Autodesk Inventor part; units mm, degrees
ref_plane "YZ Plane" through (0, 0, 0) normal (1, 0, 0) x (0, 1, 0)
ref_plane "XZ Plane" through (0, 0, 0) normal (0, 1, 0) x (-1, 0, 0)
ref_plane "XY Plane" through (0, 0, 0) normal (0, 0, 1) x (1, 0, 0)
sketch "Boceto1" plane through (0, 0, 0) normal (1, 0, 0) x (0, 1, 0)
  line L0 (-16, 16) -> (16, 16)
  line L1 (16, 16) -> (16, -16)
  line L2 (16, -16) -> (-16, -16)
  line L3 (-16, -16) -> (-16, 16)
  line L4 (-16, 16) -> (16, -16) construction
  line L5 (16, 16) -> (-16, -16) construction
  line L6 (17, 17) -> (-17, 17)
  line L7 (-17, 17) -> (-17, -17)
  line L8 (-17, -17) -> (17, -17)
  line L9 (17, -17) -> (17, 17)
  line L10 (17, 17) -> (-17, -17) construction
  line L11 (-17, 17) -> (17, -17) construction
  point P0 (0, 0)
  dimension "d0" = 32
  dimension "d1" = 32
  dimension "d2" = 34
  dimension "d3" = 34
extrude "Extrusión1" add sketch "Boceto1" along normal blind 100
sketch "Boceto5" plane through (0, 17, 17) normal (0, 1, 0) x (1, 0, 0)
  line L0 (100, 1) -> (100, 33)
  line L1 (100, 17) -> (88.5, 17) construction
  line L2 (88.5, 17) -> (82, 17) construction
  line L3 (82, 17) -> (82, 30.5) construction
  circle A0 centre (82, 30.5) radius 1.25
  circle A1 centre (74, 30.5) radius 1.25
  line L4 (80.5, 17) -> (74, 17) construction
  circle A2 centre (66, 30.5) radius 1.25
  line L5 (72.5, 17) -> (66, 17) construction
  circle A3 centre (58, 30.5) radius 1.25
  line L6 (64.5, 17) -> (58, 17) construction
  circle A4 centre (82, 3.5) radius 1.25
  line L7 (88.5, -10) -> (82, -10) construction
  circle A5 centre (74, 3.5) radius 1.25
  line L8 (80.5, -10) -> (74, -10) construction
  circle A6 centre (66, 3.5) radius 1.25
  line L9 (72.5, -10) -> (66, -10) construction
  circle A7 centre (58, 3.5) radius 1.25
  line L10 (64.5, -10) -> (58, -10) construction
  circle A8 centre (88.5, 17) radius 11.5
  point P0 (0, 17)
  dimension "d26" = 11.5
  dimension "d27" = 6.5
  dimension "d28" = 13.5
  dimension "d29" = 2.5
  dimension "d32" = 8
  dimension "d35" = 27
  dimension "d38" = 23
extrude "Extrusión4" cut sketch "Boceto5" against normal through all
sketch "Boceto6" plane through (0, 17, 17) normal (0, 1, 0) x (1, 0, 0)
  line L0 (100, 17) -> (100, 34)
  line L1 (100, 17) -> (56, 17) construction
  line L2 (0, 0) -> (100, 0)
  line L3 (56, 0) -> (56, 7) construction
  line L4 (56, 34) -> (56, 27) construction
  line L5 (56, 27) -> (56, 7)
  line L6 (56, 7) -> (83.498, 7)
  line L7 (56, 0) -> (56, 7) construction
  line L8 (56, 27) -> (83.498, 27)
  line L9 (83.498, 27) -> (83.498, 7)
  point P0 (0, 17)
  dimension "d41" = 44
  dimension "d42" = 7
extrude "Extrusión5" cut sketch "Boceto6" against normal through all
sketch "Boceto7" plane through (0, 17, 17) normal (0, 1, 0) x (1, 0, 0)
  arc A0 (100, 17) -> (82.8211, 27) centre (88.5, 17) ccw
  line L0 (88.5, 17) -> (88.5, 28.5)
  line L1 (88.5, 28.5) -> (103.9894, 28.5)
  line L2 (88.5, 17) -> (100, 17) construction
  line L3 (88.5, 17) -> (88.5, 5.5)
  line L4 (88.5, 5.5) -> (103.9894, 5.5)
  line L5 (103.9894, 28.5) -> (103.9894, 5.5)
  point P0 (0, 17)
extrude "Extrusión6" cut sketch "Boceto7" against normal through all
sketch "Boceto8" plane through (0, 17, 17) normal (0, 1, 0) x (1, 0, 0)
  line L0 (0, 17) -> (5, 17)
  dimension "d47" = 5
hole "Agujero1" at (5, 17, 0) direction (0, -1, 0) diameter 2.75 end through all
sketch "Boceto9" plane through (0, 0, 0) normal (-1, 0, 0) x (0, 0, 1)
  line L0 (-11.5, 16) -> (-16, 16)
  line L1 (11.5, -16) -> (16, -16)
  line L2 (-16, 16) -> (16, 16)
  line L3 (16, 16) -> (16, -16)
  line L4 (16, -16) -> (-16, -16)
  line L5 (-16, -16) -> (-16, 16)
  line L6 (-17, 17) -> (17, 17)
  line L7 (17, 17) -> (17, -17)
  line L8 (-17, 17) -> (17, 17)
  line L9 (17, 17) -> (17, -17)
  line L10 (17, -17) -> (-17, -17)
  line L11 (-17, -17) -> (-17, 17)
  point P0 (0, 0)
extrude "Extrusión7" add sketch "Boceto9" along normal blind 20
properties part number "Eslabon_L" material "Plástico ABS"
Geometry: final body of the model. Coordinates: model frame, mm. Coordinates: 2 decimals unless noted, no trailing zeros. Order: outer loops, then holes, each group sorted by start corner. A loop starts at its lowest first (then second) coordinate and runs counter-clockwise, first axis right, second up.
Item 1: Section query D-D (x = 5). Output: boundary loops of the cut face in (y, z) (3 decimals), then the cut area to 4 significant figures.
Answer:
outline: (-17, -17) - (17, -17) - (17, -1.375) - (16, -1.375) - (16, -16) - (-16, -16) - (-16, -1.375) - (-17, -1.375) - close; (-17, 1.375) - (-16, 1.375) - (-16, 16) - (16, 16) - (16, 1.375) - (17, 1.375) - (17, 17) - (-17, 17) - close
area: 126.5 mm2
Item 2: Draft query along X for faces 1 (the face through (75.19, -16.49, -13.88)), 2 (the face through (100, -0.1, 16.3)), 3 (the face through (41, 0, -16)). Return one class per face: released by +X, released by -X, zero draft, split by the parting line, or undercut.
Answer:
face 1: undercut
face 2: released by +X
face 3: zero draft
Item 3: Material intervals for line 1 along X through (y, z) = (-16.3, 13.5); line 2 along Z through (x, y) = (82, 16.85); line 3 along Y through (x, z) = (26, -11), sorted ascending.
Answer:
line 1: x = -20 to 56.75, 59.25 to 64.75, 67.25 to 72.75, 75.25 to 80.75, 83.25 to 100
line 2: z = -17 to -14.75, -12.25 to -10, 10 to 12.25, 14.75 to 17
line 3: y = -17 to -16, 16 to 17
Item 4: Section query B-B (x = 58). State how many separate pieces and enclosed holes the cut face has, then the cut area to 3 significant figures.
Answer:
separate pieces: 6
enclosed holes: 0
area: 82.0 mm2
Item 5: Contact query for a flat-ended pin moving along its axis: P1, Ø1.1, axis at y = -16.5, z = 0.5, coming from the +X side. Output: stop coordinate, or through.
Answer:
P1: stops at x = 56
Item 6: Section query C-C (z = 0). Output: boundary loops of the cut face in (x, y) (3 decimals).
Answer:
outline: (-20, -17) - (3.625, -17) - (3.625, -16) - (-20, -16) - close; (-20, 16) - (3.625, 16) - (3.625, 17) - (-20, 17) - close; (6.375, -17) - (56, -17) - (56, -16) - (6.375, -16) - close; (6.375, 16) - (56, 16) - (56, 17) - (6.375, 17) - close
Item 7: Section query A-A (y = -13.5). Output: boundary loops of the cut face in (x, z).
Answer:
outline: (-20, -17) - (100, -17) - (100, -16) - (-20, -16) - close; (-20, 16) - (100, 16) - (100, 17) - (-20, 17) - close
